Check sheet for the modelled part. Datum: model origin and axes. Units: mm. A direction names the side the tool comes from. Give positions to 0.01 mm unless a question says otherwise; leave off trailing zeros. Write each loop counter-clockwise with the first axis right and the second up, starting at its lowest first coordinate (ties: lowest second). Pieces come first, ordered by that corner, then holes. Notation, with made-up numbers: (24, 64) -> (71, 64) arc R20 ccw to (71, 102) -> close; hole circle Ø1 at (-8, 46). An arc over 180 degrees is marked (long way). Answer as a JSON object with one key per item and string values.
from build123d import *

# Parameters (mm, degrees)
SKETCH1_W                                           = 20
SKETCH1_H                                           = 40
BOSS_EXTRUDE1_DEPTH                                 = 5
SKETCH2_W                                           = 20
SKETCH2_H                                           = 9.75
BOSS_EXTRUDE2_DEPTH                                 = 7
SKETCH3_R                                           = 1.75
CUT_EXTRUDE1_DEPTH                                  = 26.377155081
CBORE_FOR_M3_HEX_SOCKET_HEAD_CAP_SCREW1_D           = 3.4
CBORE_FOR_M3_HEX_SOCKET_HEAD_CAP_SCREW1_CBORE_D     = 6.5
CBORE_FOR_M3_HEX_SOCKET_HEAD_CAP_SCREW1_CBORE_DEPTH = 3.4
FILLET1_R                                           = 5


with BuildPart() as part:
    # Sketch1 → Boss-Extrude1 (new body)
    with BuildSketch(Plane(origin=(0, 0, 0), x_dir=(1, 0, 0), z_dir=(0, 1, 0))):
        Rectangle(SKETCH1_W, SKETCH1_H)
    extrude(amount=BOSS_EXTRUDE1_DEPTH)

    # Sketch2 → Boss-Extrude2 (add)
    with BuildSketch(Plane(origin=(0, 5, 0), x_dir=(1, 0, 0), z_dir=(0, 1, 0))):
        with Locations((0, -15.125)):
            Rectangle(SKETCH2_W, SKETCH2_H)
        with Locations((0, 15.125)):
            Rectangle(SKETCH2_W, SKETCH2_H)
    extrude(amount=BOSS_EXTRUDE2_DEPTH)

    # Sketch3 → Cut-Extrude1 (cut, through all)
    with BuildSketch(Plane.XZ):
        with Locations(Location((5, 15, 0), (0, 0, 270))):
            Circle(SKETCH3_R)
        with Locations(Location((-5, 15, 0), (0, 0, 270))):
            Circle(SKETCH3_R)
        with Locations(Location((-5, -15, 0), (0, 0, 270))):
            Circle(SKETCH3_R)
        with Locations(Location((5, -15, 0), (0, 0, 270))):
            Circle(SKETCH3_R)
    extrude(amount=-CUT_EXTRUDE1_DEPTH, mode=Mode.SUBTRACT)

    # CBORE for M3 Hex Socket Head Cap Screw1 (through all)
    with Locations(Plane(origin=(0, 0, 0), x_dir=(-1, 0, 0), z_dir=(0, -1, 0))):
        with Locations((-5, -15), (5, -15), (5, 15), (-5, 15)):
            CounterBoreHole(CBORE_FOR_M3_HEX_SOCKET_HEAD_CAP_SCREW1_D / 2, CBORE_FOR_M3_HEX_SOCKET_HEAD_CAP_SCREW1_CBORE_D / 2, CBORE_FOR_M3_HEX_SOCKET_HEAD_CAP_SCREW1_CBORE_DEPTH)

    # Fillet1
    fillet1_edges = [part.edges().sort_by_distance(p)[0] for p in [
        (10, 6, 20),
        (-10, 6, 20),
        (-10, 6, -20),
        (10, 6, -20),
    ]]
    fillet(fillet1_edges, radius=FILLET1_R)


solid = part.part
1. Mould release check, pull along X, two halves, no side actions. Record for faces 4 (the face through (0, 8, -10.25)), 5 (the face through (-5.67, 7.64, -16.617)), 6 (the face through (-9, 6, 18)): released by +X, released by -X, zero draft, split by the parting line, or undercut.
Determined:
{"face 4": "zero draft", "face 5": "undercut", "face 6": "released by -X"}
2. Sectioned sample at D-D, the plane z = 8. Enter the section's corners in (x, y), plus the area to 3 significant figures.
Determined:
{"outline": "(-10, 0) -> (10, 0) -> (10, 5) -> (-10, 5) -> close", "area": "100 mm^2"}
3. Sectioned sample at B-B, the plane x = -6. Enter the section's corners in (y, z), plus the area to 3 significant figures.
Determined:
{"outline": "(0, -19.9) -> (12, -19.9) -> (12, -16.44) -> (3.4, -16.44) -> (3.4, -18.09) -> (0, -18.09) -> close; (0, -11.91) -> (3.4, -11.91) -> (3.4, -13.56) -> (12, -13.56) -> (12, -10.25) -> (5, -10.25) -> (5, 10.25) -> (12, 10.25) -> (12, 13.56) -> (3.4, 13.56) -> (3.4, 11.91) -> (0, 11.91) -> close; (0, 18.09) -> (3.4, 18.09) -> (3.4, 16.44) -> (12, 16.44) -> (12, 19.9) -> (0, 19.9) -> close", "area": "243 mm^2"}
4. Sectioned sample at C-C, the plane x = 0.5. Enter the section's corners in (y, z), plus the area to 4 significant figures.
Determined:
{"outline": "(0, -20) -> (12, -20) -> (12, -10.25) -> (5, -10.25) -> (5, 10.25) -> (12, 10.25) -> (12, 20) -> (0, 20) -> close", "area": "336.5 mm^2"}
5. Scan lines: L1, parallel to X at y = 9, z = 15; L2, parallel to Z at x = -5, y = 2.6; L3, parallel to X at y = 1.55, z = -15. Record each from-to range of solid material in increasing order. Write a range as [from, to].
Determined:
{"L1": "[-10, -6.75], [-3.25, 3.25], [6.75, 10]", "L2": "[-20, -18.25], [-11.75, 11.75], [18.25, 20]", "L3": "[-10, -8.25], [-1.75, 1.75], [8.25, 10]"}
6. Go/stop test with flat-tipped pins: P1, Ø5, axis at y = 9.5, z = -6, coming from the -X side; P2, Ø2, axis at x = 5.5, z = -13.5, coming from the -Y side. Record where each tip stops, or that it passes through.
Determined:
{"P1": "through", "P2": "y = 3.4"}
7. Sectioned sample at A-A, the plane y = 8.25. Enter the section's corners in (x, z), plus the area to 3 significant figures.
Determined:
{"outline": "(-10, -15) arc R5 ccw to (-5, -20) -> (5, -20) arc R5 ccw to (10, -15) -> (10, -10.25) -> (-10, -10.25) -> close; (-10, 10.25) -> (10, 10.25) -> (10, 15) arc R5 ccw to (5, 20) -> (-5, 20) arc R5 ccw to (-10, 15) -> close; hole circle Ø3.5 at (-5, -15); hole circle Ø3.5 at (-5, 15); hole circle Ø3.5 at (5, -15); hole circle Ø3.5 at (5, 15)", "area": "330 mm^2"}
8. Access from +Z, -Z, +X, -X, +Y, -Y to the whole of each face (thin tool, end or side, straight path). Record for faces 1 (the face through (-6.4, 3.4, 16.4)), 2 (the face through (0, 8, 10.25)), 3 (the face through (-10, 3, 0)).
Determined:
{"face 1": "-Y", "face 2": "+X, -X, +Y", "face 3": "+Z, -Z, -X, +Y, -Y"}
